Could you check a few things on this model? Use its own coordinates, in mm. Round coordinates to 2 decimals unless told otherwise and drop trailing zeros. Write each loop counter-clockwise with the first axis right and the second up, starting at its lowest first coordinate (ties: lowest second). Pieces come first, ordered by that corner, then holes. Notation, with made-up numbers: M 42,-13 L 66,-13 A28 cw 66,12 Z; hole C 7,60 d4. An arc over 180 degrees is marked long. One line per item, written item: value. Start each with the question number.
(1) Thinking about a two-plate mould opening in Z: for faces 1 (the face through (-1, 0, 97.5)), 2 (the face through (-1, 33, -30)), 3 (the face through (-1, 35, 20)), which applies, released by +Z, released by -Z, zero draft, split by the parting line, or undercut?
(2) I want a section at A-A on z = -8. Please give me the cut outline in (x, y).
(3) If I drill on L1, parallel to Y at x = -52.5, z = -21.5, over which ranges is the centre line in solid material (lowest first)?
```python
from build123d import *

# Parameters (mm, degrees)
ESQUISSE1_W             = 165
ESQUISSE1_H             = 195
BOSS_EXTRU_1_DEPTH      = 35
ESQUISSE4_W             = 120
ESQUISSE4_H             = 60
ENL_V_MAT_EXTRU_1_DEPTH = 2


with BuildPart() as part:
    # Esquisse1 → Boss.-Extru.1 (new body, symmetric)
    with BuildSketch(Plane(origin=(0, 0, 0), x_dir=(1, 0, 0), z_dir=(0, 1, 0))):
        Rectangle(ESQUISSE1_W, ESQUISSE1_H)
    extrude(amount=BOSS_EXTRU_1_DEPTH, both=True)

    # Esquisse4 → Enlèv. mat.-Extru.1 (cut)
    with BuildSketch(Plane(origin=(0, 35, 0), x_dir=(1, 0, 0), z_dir=(0, 1, 0))):
        with Locations((0, 30)):
            Rectangle(ESQUISSE4_W, ESQUISSE4_H)
    extrude(amount=-ENL_V_MAT_EXTRU_1_DEPTH, mode=Mode.SUBTRACT)


solid = part.part
```
Found:
1. face 1: released by +Z
1. face 2: undercut
1. face 3: zero draft
2. outline: M -82.5,-35 L 82.5,-35 L 82.5,35 L 60,35 L 60,33 L -60,33 L -60,35 L -82.5,35 Z
3. L1: y = -35 to 33
